Job drawing, mm, ordinate dimensions from the low corner. One solid piece. Coordinates: 2 decimals unless noted, no trailing zeros. Order: outer loops, then holes, each group sorted by start corner. A loop starts at its lowest first (then second) coordinate and runs counter-clockwise, first axis right, second up. Notation, with made-up numbers: M -33,77 L 21,77 A31 cw 21,109 Z; hole C -10,87 d8. An arc over 180 degrees is marked long. Write item = value, one per line.
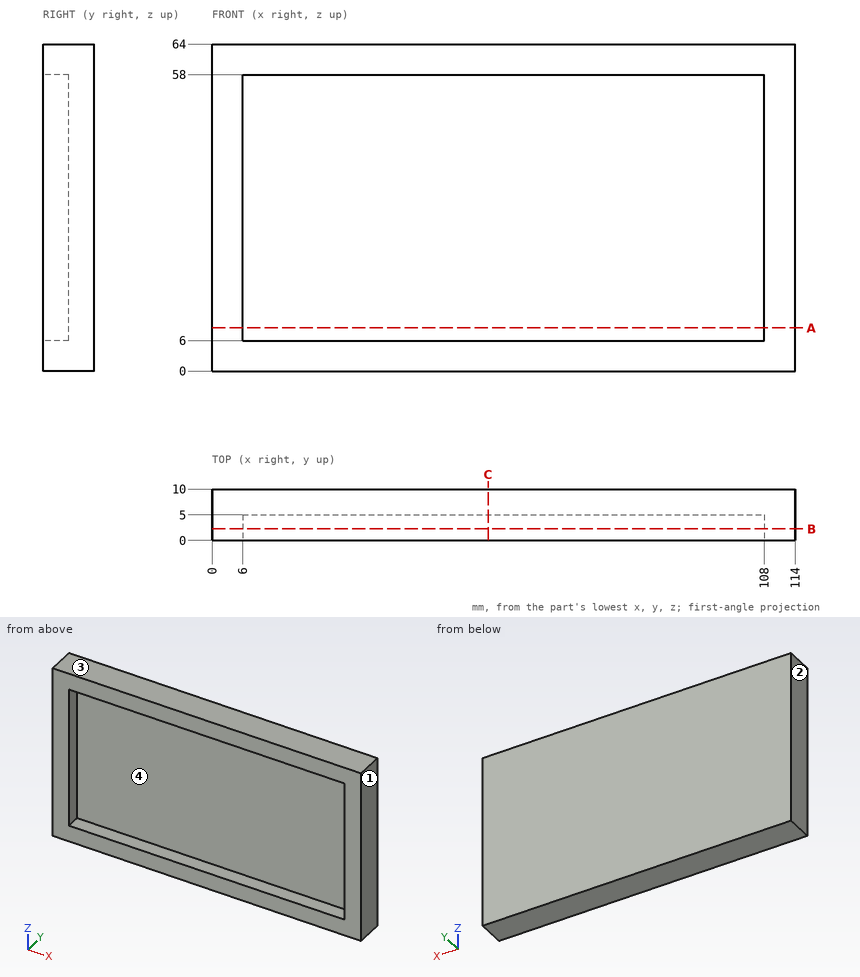
(1) Slice it at A-A, the plane z = 8.5. Write the cut outline in (x, y).
Evaluation:
outline = M 0,0 L 6,0 L 6,5 L 108,5 L 108,0 L 114,0 L 114,10 L 0,10 Z
(2) Pull direction X, two halves, no side cores. Call the marked faces 1, 2, 3 and 4: +X half, -X half, draft (parallel to the pull), parting line (faces both ways), or undercut.
Evaluation:
face_1 = +X half
face_2 = -X half
face_3 = draft
face_4 = undercut
(3) Pin check, flat tip, straight feed: pin 1 Ø2 at (x, z) = (27.5, 50.5) entering from -Y. Stop position of the tip, or through.
Evaluation:
pin_1 = 5
(4) Wall check: line 1 (X direction, y = 3.5, z = 52); line 2 (Z direction, x = 79.5, y = 2); line 3 (Y direction, x = 100.5, z = 13.5). Give the ranges that are in metal, low to high. Write a range as from..to.
Evaluation:
line_1 = 0..6, 108..114
line_2 = 0..6, 58..64
line_3 = 5..10
(5) Slice it at C-C, the plane x = 54. Write the cut outline in (y, z).
Evaluation:
outline = M 0,0 L 10,0 L 10,64 L 0,64 L 0,58 L 5,58 L 5,6 L 0,6 Z
(6) Slice it at B-B, the plane y = 2.25. Write the cut outline in (x, z), then the cut area to 3 significant figures.
Evaluation:
outline = M 0,0 L 114,0 L 114,64 L 0,64 Z; hole M 6,6 L 108,6 L 108,58 L 6,58 Z
area = 1,990 mm²
